Study the drawing (mm; zero at the part's minimum x, y, z) and answer. Round coordinates to 2 decimals unless told otherwise and drop trailing zeros. Loops run counter-clockwise (first coordinate to the right, second up) from the corner with the lowest first, then second, coordinate; pieces in that order, holes last. Notation, with made-up numbers: (27, 87.5) -> (44, 87.5) arc R24 ccw to (44, 122.5) -> close; hole circle Ø7 at (-13.75, 57.5). An arc over 180 degrees is marked (long way). Use one line per item in the form item = value.
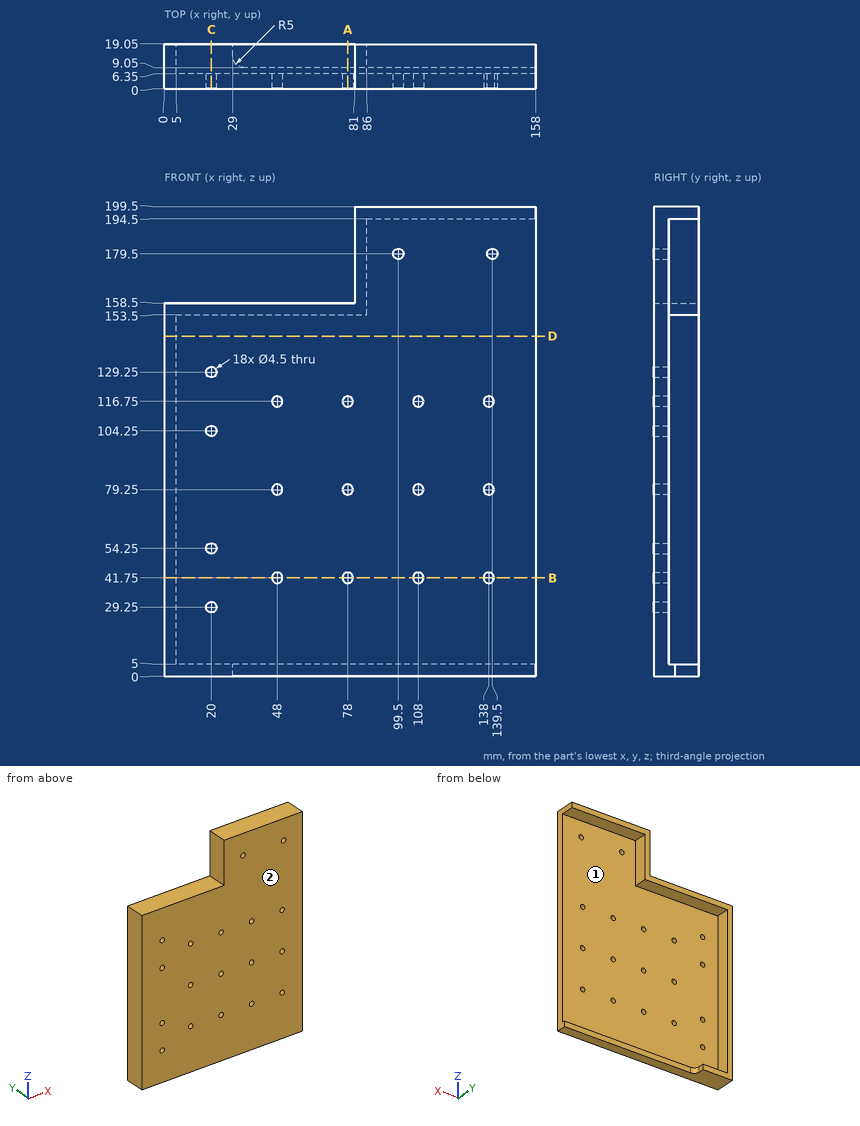
(1) Find section B-B, the plane z = 41.75. Write down the section's boundary in (x, y).
Completed:
outline = (0, 0) -> (45.75, 0) -> (45.75, 6.35) -> (5, 6.35) -> (5, 19.05) -> (0, 19.05) -> close; (50.25, 0) -> (75.75, 0) -> (75.75, 6.35) -> (50.25, 6.35) -> close; (80.25, 0) -> (105.75, 0) -> (105.75, 6.35) -> (80.25, 6.35) -> close; (110.25, 0) -> (135.75, 0) -> (135.75, 6.35) -> (110.25, 6.35) -> close; (140.25, 0) -> (158, 0) -> (158, 6.35) -> (140.25, 6.35) -> close
(2) Given P1, Ø2.5, axis at x = 138, z = 41.75, coming from the -Y side; P2, Ø6, axis at x = 96, y = 15.5, coming from the -Z side; P3, Ø4, axis at x = 38, y = 11.5, coming from the -Z side; P4, Ø7, axis at x = 20, z = 129.25, coming from the +Y side, each flat-ended and moving along its own axis, determine where each tip first touches the part or whether it passes through.
Completed:
P1 = through
P2 = 194.5
P3 = 153.5
P4 = 6.35
(3) Find section C-C, the plane x = 20. Write down the section's boundary in (y, z), then the cut area to 3 significant figures.
Completed:
outline = (0, 0) -> (19.05, 0) -> (19.05, 5) -> (6.35, 5) -> (6.35, 27) -> (0, 27) -> close; (0, 31.5) -> (6.35, 31.5) -> (6.35, 52) -> (0, 52) -> close; (0, 56.5) -> (6.35, 56.5) -> (6.35, 102) -> (0, 102) -> close; (0, 106.5) -> (6.35, 106.5) -> (6.35, 127) -> (0, 127) -> close; (0, 131.5) -> (6.35, 131.5) -> (6.35, 153.5) -> (19.05, 153.5) -> (19.05, 158.5) -> (0, 158.5) -> close
area = 1,020 mm2
(4) For a pull along Z with two mould halves and no side action, classify the marked faces 1 and 2 as +Z half, -Z half, draft (parallel to the pull), parting line (faces both ways), or undercut.
Completed:
face_1 = undercut
face_2 = draft
(5) Find section D-D, the plane z = 144.5. Write down the section's boundary in (x, y).
Completed:
outline = (0, 0) -> (158, 0) -> (158, 6.35) -> (5, 6.35) -> (5, 19.05) -> (0, 19.05) -> close
(6) Find section A-A, the plane x = 78. Write down the section's boundary in (y, z), then the cut area to 3 significant figures.
Completed:
outline = (0, 0) -> (9.05, 0) -> (9.05, 5) -> (6.35, 5) -> (6.35, 39.5) -> (0, 39.5) -> close; (0, 44) -> (6.35, 44) -> (6.35, 77) -> (0, 77) -> close; (0, 81.5) -> (6.35, 81.5) -> (6.35, 114.5) -> (0, 114.5) -> close; (0, 119) -> (6.35, 119) -> (6.35, 153.5) -> (19.05, 153.5) -> (19.05, 158.5) -> (0, 158.5) -> close
area = 998 mm2
(7) Consider L1, parallel to X at y = 2.75, z = 41.75; L2, parallel to X at y = 2.75, z = 179.5; L3, parallel to Z at x = 108, y = 2. Determine where each line is inside the solid, lowest interval first.
Completed:
L1 = 0 to 45.75, 50.25 to 75.75, 80.25 to 105.75, 110.25 to 135.75, 140.25 to 158
L2 = 81 to 97.25, 101.75 to 137.25, 141.75 to 158
L3 = 0 to 39.5, 44 to 77, 81.5 to 114.5, 119 to 199.5
